Geometry check sheet. Reference: the model listing, model coordinates, mm. A direction names the side the tool comes from. Give positions to 0.01 mm unless a question says otherwise; leave off trailing zeros. Loops run counter-clockwise (first coordinate to the right, second up) from the corner with the lowest first, then second, coordinate; pieces in that order, holes last.
1. Tool access check on faces 5 (the cylindrical face through (-153.703, 32.388, 2.504)), 6 (the cylindrical face through (-143.44, 37.88, 2.5)). Record the directions out of +Z, -Z, +X, -X, +Y, -Y that give a thin tool (end or side, any length) a straight path to the whole face; none if there is none.
2. Material ranges on L1, parallel to X at y = 58.5, z = 2; L2, parallel to X at y = 36, z = 3.65; L3, parallel to Y at x = -142.5, z = 0.7, recorded low to high.
3. Cross-section at B-B, the plane x = -141.75. Record the cut outline in (y, z).
4. Cross-section at D-D, the plane x = -134.25. Record the cut outline in (y, z).
5. Cross-section at C-C, the plane z = 2.6. Record the cut outline in (x, y).
6. Go/stop test with a flat-tipped pin: pin 1 Ø1.5 at (x, y) = (-136, 73) entering from -Z. Record where the tip stops, or that it passes through.
7. Cross-section at A-A, the plane y = 55.5. Record the cut outline in (x, z).
8. Release check for a two-part mould opening along Y. For faces 1 (the flat face through (-144, 30.939, 3)), 2 (the flat face through (-146.509, 55, 3)), 3 (the cylindrical face through (-143.58, 73.31, 2.5)), 4 (the flat face through (-149, 55, 5.08)) record: +Y half, -Y half, draft (parallel to the pull), parting line (faces both ways), or undercut.
from build123d import *

# Parameters (mm, degrees)
SKETCH1_R           = 3
BOSS_EXTRUDE1_DEPTH = 5.08


with BuildPart() as part:
    # Sketch1 → Boss-Extrude1 (new body)
    with BuildSketch(Plane.XY):
        with BuildLine():
            Line((-132.737233389, 79.19925206), (-132.737233389, 74.11925206))
            Line((-132.737233389, 74.11925206), (-132.737233389, 36.01925206))
            ThreePointArc((-132.737233389, 36.01925206), (-134.22513094, 32.427149612), (-137.817233389, 30.93925206))
            Line((-137.817233389, 30.93925206), (-150.150857378, 30.93925206))
            ThreePointArc((-150.150857378, 30.93925206), (-153.742959826, 32.427149612), (-155.230857378, 36.01925206))
            Line((-155.230857378, 36.01925206), (-155.230857378, 74.11925206))
            Line((-155.230857378, 74.11925206), (-155.230857378, 79.19925206))
            Line((-155.230857378, 79.19925206), (-132.737233389, 79.19925206))
        make_face()
        with Locations((-143.509134839, 34.161720172)):
            Circle(SKETCH1_R, mode=Mode.SUBTRACT)
        with BuildLine():
            Line((-140.509134839, 70.311824491), (-140.509134839, 40.878834509))
            ThreePointArc((-140.509134839, 40.878834509), (-143.509134839, 37.878834509), (-146.509134839, 40.878834509))
            Line((-146.509134839, 40.878834509), (-146.509134839, 70.311824491))
            ThreePointArc((-146.509134839, 70.311824491), (-143.509134839, 73.311824491), (-140.509134839, 70.311824491))
        make_face(mode=Mode.SUBTRACT)
    extrude(amount=BOSS_EXTRUDE1_DEPTH)


solid = part.part
Result:
1. face 5: +Z, -Z, -X, -Y
1. face 6: +Z, -Z
2. L1: x = -155.23 to -146.51, -140.51 to -132.74
2. L2: x = -155.23 to -145.88, -141.14 to -132.74
2. L3: y = 30.94 to 31.34, 36.99 to 38.05, 73.14 to 79.2
3. outline: (30.94, 0) - (31.73, 0) - (31.73, 5.08) - (30.94, 5.08) - close; (36.59, 0) - (38.45, 0) - (38.45, 5.08) - (36.59, 5.08) - close; (72.74, 0) - (79.2, 0) - (79.2, 5.08) - (72.74, 5.08) - close
4. outline: (32.4, 0) - (79.2, 0) - (79.2, 5.08) - (32.4, 5.08) - close
5. outline: (-155.23, 36.02) arc R5.08 ccw to (-150.15, 30.94) - (-137.82, 30.94) arc R5.08 ccw to (-132.74, 36.02) - (-132.74, 79.2) - (-155.23, 79.2) - close; hole circle Ø6 at (-143.51, 34.16); hole (-146.51, 40.88) arc R3 ccw to (-140.51, 40.88) - (-140.51, 70.31) arc R3 ccw to (-146.51, 70.31) - close
6. pin 1: stops at z = 0
7. outline: (-155.23, 0) - (-146.51, 0) - (-146.51, 5.08) - (-155.23, 5.08) - close; (-140.51, 0) - (-132.74, 0) - (-132.74, 5.08) - (-140.51, 5.08) - close
8. face 1: -Y half
8. face 2: undercut
8. face 3: undercut
8. face 4: draft
